```python
from build123d import *

# Parameters (mm, degrees)
SKETCH1_W           = 100
SKETCH1_H           = 100
BOSS_EXTRUDE1_DEPTH = 50
SKETCH3_W           = 80
SKETCH3_H           = 30
CUT_EXTRUDE2_DEPTH  = 15
FILLET1_R           = 10
SKETCH4_R           = 10
CUT_EXTRUDE3_DEPTH  = 15
SKETCH5_R           = 10
CUT_EXTRUDE4_DEPTH  = 146.688022843


with BuildPart() as part:
    # Sketch1 → Boss-Extrude1 (new body)
    with BuildSketch(Plane(origin=(0, 0, 0), x_dir=(1, 0, 0), z_dir=(0, 1, 0))):
        with Locations((50, 50)):
            Rectangle(SKETCH1_W, SKETCH1_H)
    extrude(amount=BOSS_EXTRUDE1_DEPTH)

    # Sketch3 → Cut-Extrude2 (cut)
    with BuildSketch(Plane(origin=(0, 50, 0), x_dir=(1, 0, 0), z_dir=(0, 1, 0))):
        with Locations((50, 25)):
            Rectangle(SKETCH3_W, SKETCH3_H)
    extrude(amount=-CUT_EXTRUDE2_DEPTH, mode=Mode.SUBTRACT)

    # Fillet1
    fillet1_edges = [part.edges().sort_by_distance(p)[0] for p in [
        (10, 42.5, -10),
        (10, 42.5, -40),
        (90, 42.5, -40),
        (90, 42.5, -10),
    ]]
    fillet(fillet1_edges, radius=FILLET1_R)

    # Sketch4 → Cut-Extrude3 (cut)
    with BuildSketch(Plane(origin=(0, 35, 0), x_dir=(1, 0, 0), z_dir=(0, 1, 0))):
        with Locations(Location((25, 25, 0), (0, 0, 270))):
            Circle(SKETCH4_R)
        with Locations(Location((75, 25, 0), (0, 0, 270))):
            Circle(SKETCH4_R)
    extrude(amount=-CUT_EXTRUDE3_DEPTH, mode=Mode.SUBTRACT)

    # Sketch5 → Cut-Extrude4 (cut, through all)
    with BuildSketch(Plane(origin=(0, 35, 0), x_dir=(1, 0, 0), z_dir=(0, 1, 0))):
        with Locations(Location((50, 25, 0), (0, 0, 270))):
            Circle(SKETCH5_R)
    extrude(amount=-CUT_EXTRUDE4_DEPTH, mode=Mode.SUBTRACT)


solid = part.part
```
Geometry check sheet. Reference: the model listing, model coordinates, mm. A direction names the side the tool comes from. Coordinates: 2 decimals unless noted, no trailing zeros. Loops run counter-clockwise (first coordinate to the right, second up) from the corner with the lowest first, then second, coordinate; pieces in that order, holes last. Notation, with made-up numbers: (-26, -39) -> (15, -39) arc R11 cw to (15, -24) -> close; hole circle Ø8 at (-26, 53.25). An arc over 180 degrees is marked (long way). Put each result on its own line as item: value.
1) Tool access check on faces 1 (the flat face through (100, 25, -49)), 2 (the flat face through (90, 43, -25)). Record the directions out of +Z, -Z, +X, -X, +Y, -Y that give a thin tool (end or side, any length) a straight path to the whole face; none if there is none.
Result set:
face 1: +Z, -Z, +X, +Y, -Y
face 2: +Y
2) Gauge pin test, flat ends, axial feed: pin 1 Ø16 at (x, z) = (77, -24.5) entering from +Y; pin 2 Ø16 at (x, z) = (25, -25) entering from +Y. Record the tip position at first contact, or that the pin passes through.
Result set:
pin 1: stops at y = 35
pin 2: stops at y = 20
3) Cross-section at A-A on x = 56. Record the boundary of the cut face in (y, z).
Result set:
outline: (0, -100) -> (50, -100) -> (50, -40) -> (35, -40) -> (35, -33) -> (0, -33) -> close; (0, -17) -> (35, -17) -> (35, -10) -> (50, -10) -> (50, 0) -> (0, 0) -> close
4) Release check for a two-part mould opening along Z. For faces 3 (the cylindrical face through (41.128, 17.745, -20.386)), 4 (the flat face through (49, 25, 0)), 5 (the flat face through (49, 50, -62)) record: released by +Z, released by -Z, zero draft, split by the parting line, or undercut.
Result set:
face 3: undercut
face 4: released by +Z
face 5: zero draft
5) Cross-section at B-B on y = 9. Record the boundary of the cut face in (x, z).
Result set:
outline: (0, -100) -> (100, -100) -> (100, 0) -> (0, 0) -> close; hole circle Ø20 at (50, -25)
6) Cross-section at D-D on y = 42. Record the boundary of the cut face in (x, z), plus the area to 3 significant figures.
Result set:
outline: (0, -100) -> (100, -100) -> (100, 0) -> (0, 0) -> close; hole (10, -30) arc R10 ccw to (20, -40) -> (80, -40) arc R10 ccw to (90, -30) -> (90, -20) arc R10 ccw to (80, -10) -> (20, -10) arc R10 ccw to (10, -20) -> close
area: 7,690 mm^2
7) Thickness scan on line 1 (X direction, y = 28, z = -25); line 2 (Z direction, x = 73.5, y = 43); line 3 (Z direction, x = 52, y = 5.5). Record the ranges inside material, lowest first.
Result set:
line 1: x = 0 to 15, 35 to 40, 60 to 65, 85 to 100
line 2: z = -100 to -40, -10 to 0
line 3: z = -100 to -34.8, -15.2 to 0
8) Cross-section at C-C on x = 12. Record the boundary of the cut face in (y, z), plus the area to 3 significant figures.
Result set:
outline: (0, -100) -> (50, -100) -> (50, -36) -> (35, -36) -> (35, -14) -> (50, -14) -> (50, 0) -> (0, 0) -> close
area: 4,670 mm^2
